Input: dimensioned drawing with shaded views. Units: mm. Origin: part minimum x, y, z. A direction names the side the tool comes from. Coordinates: 2 decimals unless noted, no trailing zeros. Put each result on its own line as item: value. Start each with the question number.
1) Reachability of the marked faces 1, 2 and 3 from +Z, -Z, +X, -X, +Y, -Y: full face, straight path, thin tool, end or side. Return the list, or none.
2) Contact query for flat-ended pins moving along their axis: pin 1 Ø1.4 at (x, y) = (60, 58.5) entering from +Z (3 decimals); pin 2 Ø10 at (x, z) = (71, 39.5) entering from -Y; pin 3 Ø10 at (x, y) = (50, 67) entering from +Z; pin 4 Ø15 at (x, y) = (94.53, 12.7) entering from -Z. Output: stop coordinate, or through.
3) Material intervals for line 1 along X through (y, z) = (12, 2) (1 decimal); line 2 along Z through (x, y) = (28, 73) (1 decimal); line 3 along Y through (x, z) = (52, 50.5) (1 decimal), sorted ascending. Write a range as from..to.
4) Section A-A on y = 50.8. Count the separate pieces of the cut face and the enclosed holes in it, and give its area (3 significant figures).
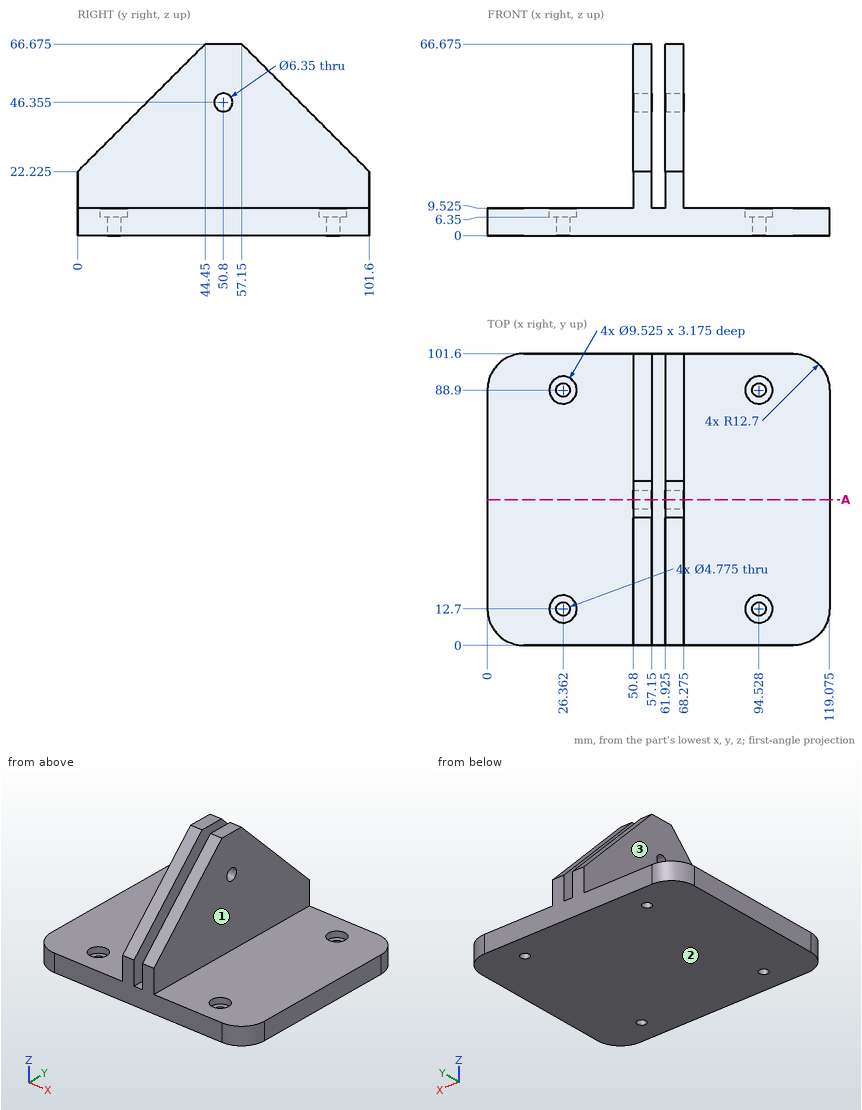
Answer block:
1. face 1: +Z, +X, +Y, -Y
1. face 2: -Z, +X, -X, +Y, -Y
1. face 3: +Z, -X, +Y, -Y
2. pin 1: stops at z = 9.525
2. pin 2: stops at y = 13.08
2. pin 3: stops at z = 61.76
2. pin 4: stops at z = 0
3. line 1: x = 0..24.1, 28.6..92.2, 96.8..119.1
3. line 2: z = 0..9.5
3. line 3: y = 28.3..73.3
4. separate pieces: 3
4. enclosed holes: 0
4. area: 1,780 mm²
